Geometry: see drawing. Coordinates: mm, zero at the bounding-box minimum. A direction names the side the tool comes from. Coordinates: 2 decimals unless noted, no trailing zeros. Loops run counter-clockwise (first coordinate to the right, second up) from the corner with the lowest first, then second, coordinate; pieces in that order, holes last.
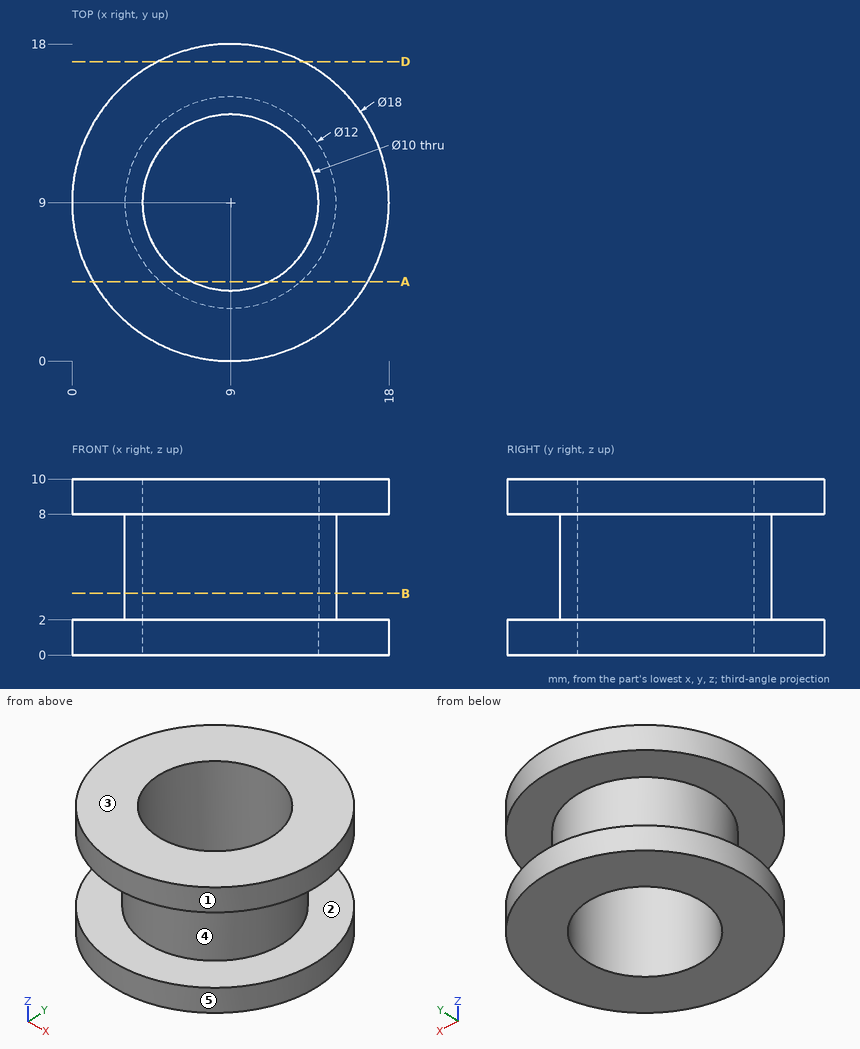
Item 1: Mould query, pull axis Z, two halves, no side actions, for the marked faces 1, 2 and 3. Classes: +Z half, -Z half, draft (parallel to the pull), parting line (faces both ways), or undercut.
Result:
face 1: draft
face 2: undercut
face 3: +Z half
Item 2: Section query A-A (y = 4.5). Output: boundary loops of the cut face in (x, z).
Result:
outline: (1.21, 0) - (6.82, 0) - (6.82, 10) - (1.21, 10) - (1.21, 8) - (5.03, 8) - (5.03, 2) - (1.21, 2) - close; (11.18, 0) - (16.79, 0) - (16.79, 2) - (12.97, 2) - (12.97, 8) - (16.79, 8) - (16.79, 10) - (11.18, 10) - close
Item 3: Section query B-B (z = 3.5). Output: boundary loops of the cut face in (x, y).
Result:
outline: circle Ø12 at (9, 9); hole circle Ø10 at (9, 9)
Item 4: Section query D-D (y = 17). Output: boundary loops of the cut face in (x, z), then the cut area to 3 significant figures.
Result:
outline: (4.88, 0) - (13.12, 0) - (13.12, 2) - (4.88, 2) - close; (4.88, 8) - (13.12, 8) - (13.12, 10) - (4.88, 10) - close
area: 33.0 mm2
Item 5: Reachability of the marked faces 4 and 5 from +Z, -Z, +X, -X, +Y, -Y: full face, straight path, thin tool, end or side. Return the list, or none.
Result:
face 4: none
face 5: +Z, -Z
Item 6: Contact query for flat-ended pins moving along their axis: P1, Ø3, axis at y = 14, z = 5, coming from the -X side; P2, Ø6, axis at x = 13, z = 8, coming from the -Y side; P3, Ø1.5, axis at x = 15, z = 1.5, coming from the +Y side. Output: stop coordinate, or through.
Result:
P1: stops at x = 4.13
P2: stops at y = 0.06
P3: stops at y = 16.31
Item 7: Line query: L1, parallel to X at y = 9, z = 5; L2, parallel to Z at x = 2.5, y = 11.75. Output: solid intervals per line, ascending.
Result:
L1: x = 3 to 4, 14 to 15
L2: z = 0 to 2, 8 to 10
